Solid Edge part; units mm, degrees
sketch "Sketch1" plane through (0, 0, 0) normal (0, -1, 0) x (1, 0, 0)
  circle A0 centre (0, 0) radius 10
extrude "Protrusion1" add sketch "Sketch1" along normal mid plane 15
sketch "Sketch2" plane through (0, 0, 0) normal (0, -1, 0) x (1, 0, 0)
  circle A0 centre (0, 0) radius 12.5
  circle A1 centre (0, 0) radius 10
extrude "ExtrudedProtrusion_3" add sketch "Sketch2" along normal mid plane 16
sketch "Sketch3" plane through (0, -7.5, 0) normal (0, -1, 0) x (1, 0, 0)
  circle A0 centre (0, 0) radius 2.5
extrude "ExtrudedCutout_1" cut sketch "Sketch3" against normal blind 20.7581
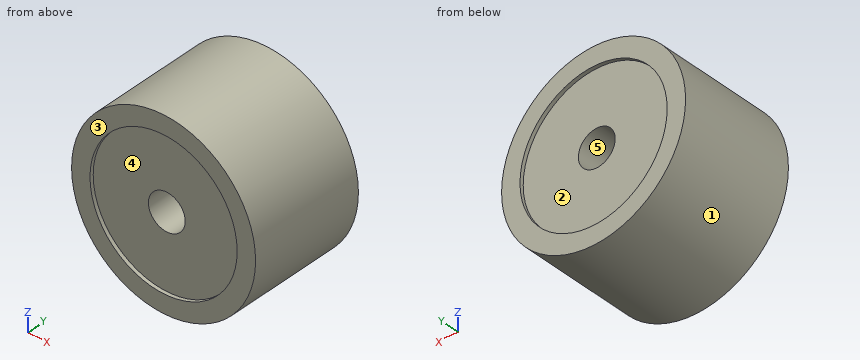
Geometry: final body of the model. Coordinates: model frame, mm. Face numbers are marked on the shaded views. A direction names the side the tool comes from. Coordinates: 2 decimals unless noted, no trailing zeros. Order: outer loops, then holes, each group sorted by start corner. A loop starts at its lowest first (then second) coordinate and runs counter-clockwise, first axis right, second up. Notation, with made-up numbers: (37, 82) - (85, 82) arc R9 cw to (85, 87) - close; hole circle Ø10 at (21.5, 35.5). An arc over 180 degrees is marked (long way). Use one line per item in the form item = value.
1) Section B-B (x = 0). Return loops of the section in (y, z).
Solutions:
outline = (-8, -12.5) - (8, -12.5) - (8, -10) - (7.5, -10) - (7.5, -2.5) - (-7.5, -2.5) - (-7.5, -10) - (-8, -10) - close; (-8, 10) - (-7.5, 10) - (-7.5, 2.5) - (7.5, 2.5) - (7.5, 10) - (8, 10) - (8, 12.5) - (-8, 12.5) - close
2) Mould query, pull axis X, two halves, no side actions, for the marked faces 1, 2 and 3. Classes: +X half, -X half, draft (parallel to the pull), parting line (faces both ways), or undercut.
Solutions:
face_1 = parting line
face_2 = undercut
face_3 = draft
3) Section A-A (z = 0). Return loops of the section in (x, y).
Solutions:
outline = (-12.5, -8) - (-10, -8) - (-10, -7.5) - (-2.5, -7.5) - (-2.5, 7.5) - (-10, 7.5) - (-10, 8) - (-12.5, 8) - close; (2.5, -7.5) - (10, -7.5) - (10, -8) - (12.5, -8) - (12.5, 8) - (10, 8) - (10, 7.5) - (2.5, 7.5) - close
4) Section C-C (y = 2.25). Return loops of the section in (x, z).
Solutions:
outline = circle Ø25 at (0, 0); hole circle Ø5 at (0, 0)
5) Set-up query: the marked faces 4 and 5. Return all of +Z, -Z, +X, -X, +Y, -Y with unobstructed straight access to the full face (end or side cutting, diameter ignored); none if empty.
Solutions:
face_4 = -Y
face_5 = +Y, -Y
6) Pin query (flat end, axial travel): pin 1 (10 mm diameter, centred on x = 4, z = -2.5, fed in from -Y); pin 2 (6 mm diameter, centred on x = 6.5, y = -2, fed in from -Z); pin 3 (4 mm diameter, centred on y = 4, z = -7.5, fed in from +X) (3 decimals). Return the tip coordinate at first contact, or that it passes through.
Solutions:
pin_1 = -7.5
pin_2 = -12
pin_3 = 11.225
7) Ray query, L1, parallel to Z at x = 0, y = 7.85; L2, parallel to Y at x = 4.5, z = -2.75; L3, parallel to X at y = -3.5, z = 2. Return the intervals inside material, ascending.
Solutions:
L1 = -12.5 to -10, 10 to 12.5
L2 = -7.5 to 7.5
L3 = -12.34 to -1.5, 1.5 to 12.34
8) Section D-D (x = -8.25). Return loops of the section in (y, z).
Solutions:
outline = (-8, -9.39) - (8, -9.39) - (8, -5.65) - (7.5, -5.65) - (7.5, 5.65) - (8, 5.65) - (8, 9.39) - (-8, 9.39) - (-8, 5.65) - (-7.5, 5.65) - (-7.5, -5.65) - (-8, -5.65) - close
